The drawing under review shows one solid part. Ordinate dimensions are in mm from its lowest x, y, z. A direction names the side the tool comes from. Give positions to 0.01 mm unless a question says otherwise; leave off trailing zeros. Loops run counter-clockwise (first coordinate to the right, second up) from the corner with the lowest first, then second, coordinate; pieces in that order, holes last. Notation, with made-up numbers: (-34, -31) - (20, -31) arc R25 cw to (20, -3) - close; hole circle Ø11 at (-35.75, 82). An arc over 180 degrees is marked (long way). Answer as CSV lines item,"result".
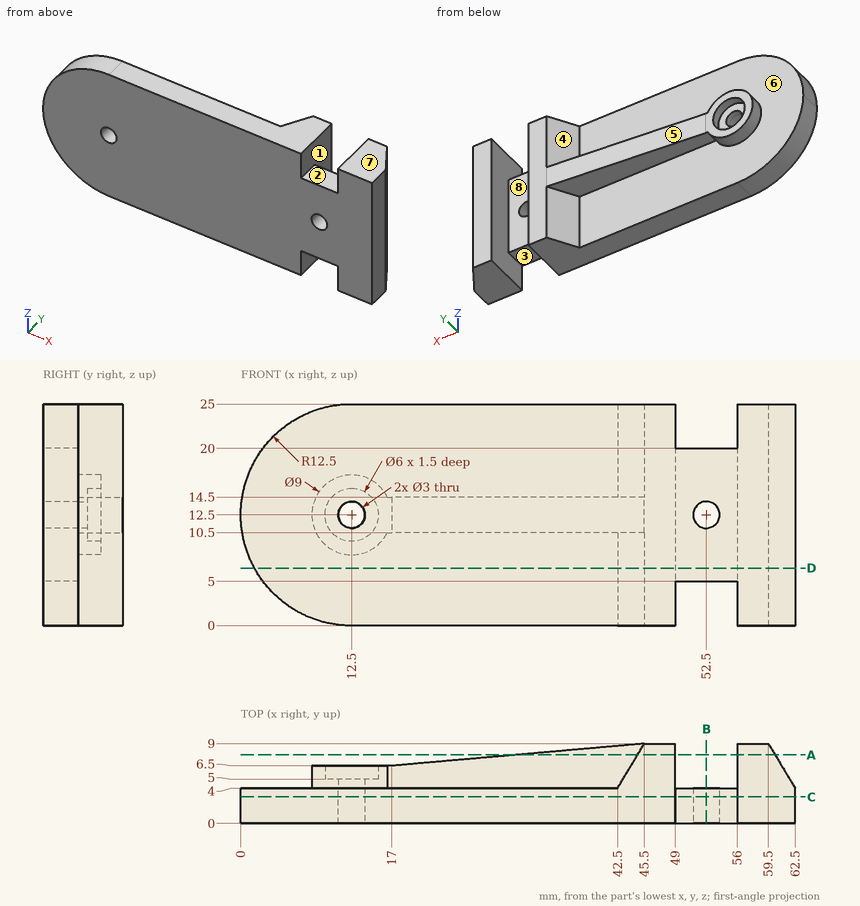
1) Machinability: for the marked faces 1, 2, 3 and 4, which of the approach directions +Z, -Z, +X, -X, +Y, -Y give a long, thin tool a straight path to every point of the face, cutting with its end or side? Answer none if there is none.
From the geometry:
face 1,"+Y"
face 2,"+Z, +Y, -Y"
face 3,"-Z, +Y, -Y"
face 4,"+Z, +Y"
2) Consider section D-D on z = 6.5. Write out the cut boundary in (x, y).
From the geometry:
outline,"(1.53, 0) - (62.5, 0) - (62.5, 4) - (59.5, 9) - (56, 9) - (56, 4) - (49, 4) - (49, 9) - (45.5, 9) - (42.5, 4) - (1.53, 4) - close"
3) Consider section A-A on y = 7.75. Write out the cut boundary in (x, z).
From the geometry:
outline,"(31.25, 10.5) - (44.75, 10.5) - (44.75, 0) - (49, 0) - (49, 25) - (44.75, 25) - (44.75, 14.5) - (31.25, 14.5) - close; (56, 0) - (60.25, 0) - (60.25, 25) - (56, 25) - close"
4) Consider section B-B on x = 52.5. Write out the cut boundary in (y, z), and give its area (3 significant figures).
From the geometry:
outline,"(0, 5) - (4, 5) - (4, 11) - (0, 11) - close; (0, 14) - (4, 14) - (4, 20) - (0, 20) - close"
area,"48.0 mm^2"
5) Wall thickness on line 1 (X direction, y = 1, z = 13.5); line 2 (Z direction, x = 55.5, y = 2.75); line 3 (X direction, y = 4.5, z = 23.75): over which ranges is each line inside the solid? List them lowest first. Write a range as from..to.
From the geometry:
line 1,"x = 0.04..11.38, 13.62..51.38, 53.62..62.5"
line 2,"z = 5..20"
line 3,"x = 42.8..49, 56..62.2"
6) Consider section C-C on y = 3. Write out the cut boundary in (x, z), and give its area (3 significant figures).
From the geometry:
outline,"(12.5, 0) - (49, 0) - (49, 5) - (56, 5) - (56, 0) - (62.5, 0) - (62.5, 25) - (56, 25) - (56, 20) - (49, 20) - (49, 25) - (12.5, 25) arc R12.5 ccw to start; hole circle Ø3 at (12.5, 12.5); hole circle Ø3 at (52.5, 12.5)"
area,"1,410 mm^2"
7) Insertion check: P1, Ø10, axis at x = 13, z = 13, coming from the +Y side; P2, Ø5.5, axis at x = 52.5, z = 16, coming from the +Y side; P3, Ø4.5, axis at y = 3, z = 15.5, coming from the -X side; P4, Ø2.5, axis at x = 12.5, z = 12.5, coming from the +Y side. Each pin has a flat end and moves straight along its axis. Give the tip position at first contact, or say it passes through.
From the geometry:
P1,"stops at y = 6.59"
P2,"stops at y = 4"
P3,"stops at x = 0.02"
P4,"passes through"
8) Draft analysis for pull direction X (two halves, no side actions). For the marked faces 5, 6, 7 and 8, state which applies: pulls with the +X half, pulls with the -X half, needs draft (parallel to the pull), parting line crosses it, or undercut.
From the geometry:
face 5,"pulls with the -X half"
face 6,"undercut"
face 7,"needs draft"
face 8,"undercut"
